Here's how the part is built. I have some questions about the finished solid (model axes, mm). A direction names the side the tool comes from. Give positions to 0.01 mm unless a question says otherwise; leave off trailing zeros. Loops run counter-clockwise (first coordinate to the right, second up) from the corner with the lowest first, then second, coordinate; pieces in that order, holes last. Notation, with made-up numbers: M 41.5,20 L 78.5,20 A16 ccw 78.5,40 Z; hole C 70.25,17 d8. An arc over 180 degrees is marked long. Answer as CSV lines item,"result". Start each with the question number.
Item 1: I want a section at B-B on z = -6. List the corners of the cut face in (x, y) for me.
Item 2: If I drill on line 1 along Z through (x, y) = (0, 7); line 2 along X through (y, z) = (48, 1); line 3 along Z through (x, y) = (2, 47.5), over which ranges is the centre line in solid material (lowest first)? Write a range as from..to.
Item 3: I want a section at A-A on y = 15.5. List the corners of the cut face in (x, z) for me.
Item 4: Will these pins go through, and if not, where does the flat tip stop? P1, Ø5.5, axis at x = 0, z = 0, coming from the +Y side; P2, Ø1, axis at x = 3, y = 45, coming from the +Z side; P3, Ø5, axis at y = 22, z = 4, coming from the -X side.
Item 5: I want a section at C-C on y = 32. List the corners of the cut face in (x, z) for me.
Item 6: If we mould it in two halves opening along X, with no side actions, what happens to faces 1 (the flat face through (-2, 0, -3)), 2 (the cylindrical face through (1.27, 10.14, -3.07)), 3 (the cylindrical face through (7.493, 29.58, -0.33)), 4 (the conical face through (0.17, 21.65, -0.55))? For each: released by +X, released by -X, zero draft, split by the parting line, or undercut.
Item 7: For faces 5 (the flat face through (-2, 60, -3)), 6 (the cylindrical face through (1.27, 49.86, 3.07)), which set-ups out of +Z, -Z, +X, -X, +Y, -Y let a thin tool reach every point of the face, with its end or its side?
Item 8: I want a section at D-D on x = 5.25. List the corners of the cut face in (y, z) for me, plus the area to 3 significant figures.
Autodesk Inventor part; units mm, degrees
ref_plane "YZ Plane" through (0, 0, 0) normal (1, 0, 0) x (0, 1, 0)
ref_plane "XZ Plane" through (0, 0, 0) normal (0, 1, 0) x (-1, 0, 0)
ref_plane "XY Plane" through (0, 0, 0) normal (0, 0, 1) x (1, 0, 0)
sketch "Sketch1" plane through (0, 0, 0) normal (0, 1, 0) x (-1, 0, 0)
  circle A0 centre (0, 0) radius 7.5
  dimension "d0" = 15
extrude "Extrusion1" add sketch "Sketch1" along normal blind 60
sketch "Sketch2" plane through (0, 60, 0) normal (0, 1, 0) x (1, 0, 0)
  circle A0 centre (0, 0) radius 7.5
sketch "Sketch3" plane through (0, 0, 0) normal (0, -1, 0) x (1, 0, 0)
  point P0 (0, 0)
  point P1 (0, 0)
hole "Hole1" at (0, 60, 0) direction (0, -1, 0) diameter 6.647 depth 20 tip angle 118
hole "Hole2" at (0, 0, 0) direction (0, 1, 0) diameter 6.647 depth 20 tip angle 118
properties part number "Support_bar"
Result:
1,outline,"M -4.5,0 L 4.5,0 L 4.5,60 L -4.5,60 Z"
2,line 1,"-7.5..-3.32, 3.32..7.5"
2,line 2,"-7.43..-3.17, 3.17..7.43"
2,line 3,"-7.23..-2.65, 2.65..7.23"
3,outline,"C 0,0 d15; hole C 0,0 d6.65"
4,P1,"y = 39.66"
4,P2,"z = 7.07"
4,P3,"x = -7.35"
5,outline,"C 0,0 d15"
6,face 1,"zero draft"
6,face 2,"undercut"
6,face 3,"split by the parting line"
6,face 4,"undercut"
7,face 5,"+Z, -Z, +X, -X, +Y"
7,face 6,"+Y"
8,outline,"M 0,-5.36 L 60,-5.36 L 60,5.36 L 0,5.36 Z"
8,area,"643 mm^2"
